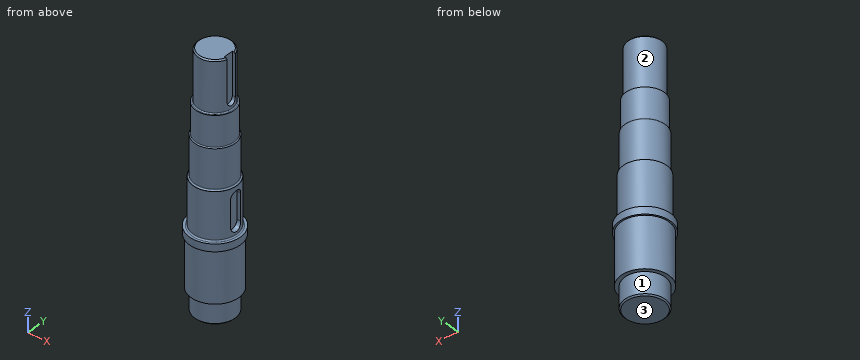
```python
from build123d import *

# Parameters (mm, degrees)
SKETCH_1_R          = 32.5
EXTRUDE_1_DEPTH     = 36
SKETCH_2_R          = 38.5
EXTRUDE_2_DEPTH     = 82
SKETCH_3_R          = 41
EXTRUDE_3_DEPTH     = 12
SKETCH_4_R          = 35
EXTRUDE_4_DEPTH     = 76
SKETCH_5_R          = 32.5
EXTRUDE_5_DEPTH     = 64
SKETCH_6_R          = 31
EXTRUDE_6_DEPTH     = 50
SKETCH_7_R          = 27.5
EXTRUDE_7_DEPTH     = 82
FILLET_1_R          = 2
FILLET_2_R          = 1.6
CHAMFER_1_SIZE      = 2
CUT_EXTRUDE_1_DEPTH = 29
CUT_EXTRUDE_2_DEPTH = 20


with BuildPart() as part:
    # 草图1 → 凸台-拉伸1 (new body)
    with BuildSketch(Plane.XY):
        Circle(SKETCH_1_R)
    extrude(amount=EXTRUDE_1_DEPTH)

    # 草图2 → 凸台-拉伸2 (add)
    with BuildSketch(Plane.XY.offset(36)):
        Circle(SKETCH_2_R)
    extrude(amount=EXTRUDE_2_DEPTH)

    # 草图3 → 凸台-拉伸3 (add)
    with BuildSketch(Plane.XY.offset(118)):
        Circle(SKETCH_3_R)
    extrude(amount=EXTRUDE_3_DEPTH)

    # 草图4 → 凸台-拉伸4 (add)
    with BuildSketch(Plane.XY.offset(130)):
        Circle(SKETCH_4_R)
    extrude(amount=EXTRUDE_4_DEPTH)

    # 草图5 → 凸台-拉伸5 (add)
    with BuildSketch(Plane.XY.offset(206)):
        Circle(SKETCH_5_R)
    extrude(amount=EXTRUDE_5_DEPTH)

    # 草图6 → 凸台-拉伸6 (add)
    with BuildSketch(Plane.XY.offset(270)):
        Circle(SKETCH_6_R)
    extrude(amount=EXTRUDE_6_DEPTH)

    # 草图7 → 凸台-拉伸7 (add)
    with BuildSketch(Plane.XY.offset(320)):
        Circle(SKETCH_7_R)
    extrude(amount=EXTRUDE_7_DEPTH)

    # 圆角1
    fillet_1_edges = [part.edges().sort_by_distance(p)[0] for p in [
        (-35, 0, 130),
        (-32.5, 0, 206),
    ]]
    fillet(fillet_1_edges, radius=FILLET_1_R)

    # 圆角2
    # the kernel refuses this fillet: 1.6 mm, written as the material it adds along each edge
    with BuildSketch(Plane(origin=(0, 0, 270), x_dir=(1, 0, 0), z_dir=(0, -1, 0))) as fillet_2_piece_1:
        with BuildLine():
            CenterArc((32.6, 1.596871942), FILLET_2_R, 180, 86.416678302)
            Line((31, 1.596871942), (30.968, 1.596871942))
            Line((30.968, 1.596871942), (30.968, 0))
            Line((30.968, 0), (31, -0.032))
            ThreePointArc((31, -0.032), (31.75, -0.032), (32.498, -0.031937439))
            Line((32.498, -0.031937439), (32.5, 0))
        make_face()
    revolve(axis=Axis((0, 0, 270), (0, 0, 1)))
    with BuildSketch(Plane(origin=(0, 0, 320), x_dir=(1, 0, 0), z_dir=(0, -1, 0))) as fillet_2_piece_2:
        with BuildLine():
            CenterArc((27.5 + FILLET_2_R, FILLET_2_R), FILLET_2_R, 180, 90)
            Line((27.5, FILLET_2_R), (27.5 - FILLET_2_R * 0.02, FILLET_2_R))
            Line((27.5 - FILLET_2_R * 0.02, FILLET_2_R), (27.5 - FILLET_2_R * 0.02, -FILLET_2_R * 0.02))
            Line((27.5 - FILLET_2_R * 0.02, -FILLET_2_R * 0.02), (27.5 + FILLET_2_R, -FILLET_2_R * 0.02))
            Line((27.5 + FILLET_2_R, -FILLET_2_R * 0.02), (27.5 + FILLET_2_R, 0))
        make_face()
    revolve(axis=Axis((0, 0, 320), (0, 0, 1)))

    # 倒角1
    chamfer_1_edges = [part.edges().sort_by_distance(p)[0] for p in [
        (-32.5, 0, 0),
        (-27.5, 0, 402),
    ]]
    chamfer(chamfer_1_edges, length=CHAMFER_1_SIZE)

    # 草图8 → 切除-拉伸1 (cut)
    with BuildSketch(Plane(origin=(27.5, 0, 0), x_dir=(0, 0, -1), z_dir=(1, 0, 0))):
        with BuildLine():
            Line((-189, 10), (-146, 10))
            ThreePointArc((-146, 10), (-136, 0), (-146, -10))
            Line((-146, -10), (-189, -10))
            ThreePointArc((-189, -10), (-199, 0), (-189, 10))
        make_face()
    extrude(amount=CUT_EXTRUDE_1_DEPTH, mode=Mode.SUBTRACT)

    # 草图9 → 切除-拉伸2 (cut)
    with BuildSketch(Plane(origin=(21.5, 0, 0), x_dir=(0, 0, -1), z_dir=(1, 0, 0))):
        with BuildLine():
            Line((-402, 8), (-334, 8))
            ThreePointArc((-334, 8), (-326, 0), (-334, -8))
            Line((-334, -8), (-402, -8))
            Line((-402, -8), (-402, 8))
        make_face()
    extrude(amount=CUT_EXTRUDE_2_DEPTH, mode=Mode.SUBTRACT)


solid = part.part
```
For this review, take the finished solid that the model builds, in its own axes (mm). Face numbers are marked on the shaded views. A direction names the side the tool comes from. Round coordinates to 2 decimals unless told otherwise and drop trailing zeros. Order: outer loops, then holes, each group sorted by start corner. A loop starts at its lowest first (then second) coordinate and runs counter-clockwise, first axis right, second up. Notation, with made-up numbers: (47.25, 77) -> (86.25, 77) arc R24 ccw to (86.25, 87) -> close; hole circle Ø6 at (16.25, 27.5). An arc over 180 degrees is marked (long way). Use a Markdown table: item, result.
Item 1: For line 1 along Z through (x, y) = (-11, 35); line 2 along X through (y, z) = (1, 180.5); line 3 along Y through (x, z) = (-0.5, 228), list the stretches that pass through material, from the lowest coordinate up. Write a range as [from, to].
Resolved:
| item | result |
|---|---|
| line 1 | z = [36, 130.02] |
| line 2 | x = [-34.99, 27.5] |
| line 3 | y = [-32.5, 32.5] |
Item 2: Machinability: for the marked faces 1, 2 and 3, which of the approach directions +Z, -Z, +X, -X, +Y, -Y give a long, thin tool a straight path to every point of the face, cutting with its end or side? Answer none if there is none.
Resolved:
| item | result |
|---|---|
| face 1 | -Z |
| face 2 | +Z |
| face 3 | -Z, +X, -X, +Y, -Y |
Item 3: Take a section at B-B (z = 168). State the section outline as (x, y) points.
Resolved:
| item | result |
|---|---|
| outline | (27.5, -10) -> (27.5, 10) -> (33.54, 10) arc R35 ccw (long way) to (33.54, -10) -> close |
Item 4: Take a section at A-A (z = 315). State the section outline as (x, y) points, plus the area to 3 significant figures.
Resolved:
| item | result |
|---|---|
| outline | circle Ø62 at (0, 0) |
| area | 3,020 mm² |
Item 5: For pin 1 (17.5 mm diameter, centred on y = -0.5, z = 347.5, fed in from +X); pin 2 (1.5 mm diameter, centred on y = 17.5, z = 228.5, fed in from -X); pin 3 (5 mm diameter, centred on x = -23, z = 183, fed in from +Y); pin 4 (23 mm diameter, centred on x = 1, y = -17.5, fed in from -Z), all flat-tipped, find the tip position at first contact; note any pin that passes through.
Resolved:
| item | result |
|---|---|
| pin 1 | stops at x = 26.31 |
| pin 2 | stops at x = -27.85 |
| pin 3 | stops at y = 28.37 |
| pin 4 | stops at z = 0 |
